Check sheet for the modelled part. Datum: model origin and axes. Units: mm. Face numbers are marked on the shaded views. A direction names the side the tool comes from. Give positions to 0.01 mm unless a question says otherwise; leave off trailing zeros. Write each loop counter-clockwise with the first axis right and the second up, starting at its lowest first coordinate (ties: lowest second). Pieces come first, ordered by that corner, then holes. Notation, with made-up numbers: M 83,89 L 131,89 A19 ccw 131,94 Z; hole C 17,51 d7. An arc over 180 degrees is marked long. Write item = value, one per line. Start each with the question number.
1) Sectioned sample at C-C, the plane z = 23. Record the cut outline in (x, y), then the cut area to 3 significant figures.
2) Gauge pin test, flat ends, axial feed: pin 1 (1 mm diameter, centred on y = 19, z = 24, fed in from +X); pin 2 (5 mm diameter, centred on x = 19, z = 14, fed in from +Y); pin 3 (10 mm diameter, centred on x = 25.5, z = 14.5, fed in from -Y). Record the tip position at first contact, or that the pin passes through.
3) Sectioned sample at A-A, the plane y = 1.75. Record the cut outline in (x, z).
4) Sectioned sample at D-D, the plane x = 2. Record the cut outline in (y, z).
5) Set-up check for the marked faces 1, 2 and 3: record each of +Z, -Z, +X, -X, +Y, -Y from which the full face is reachable in a straight line by a thin tool's end or side.
6) Draft check along X on the marked faces 4, 5 and 6. Enter one of: pulls with the +X half, pulls with the -X half, needs draft (parallel to the pull), parting line crosses it, or undercut.
7) Sectioned sample at B-B, the plane y = 8.75. Record the cut outline in (x, z), then the cut area to 3 significant figures.
8) Scan lines: L1, parallel to X at y = 13.5, z = 8.5; L2, parallel to X at y = 3.75, z = 3.5; L3, parallel to X at y = 19.75, z = 2. Record each from-to range of solid material in increasing order.
from build123d import *

# Parameters (mm, degrees)
F1_DEPTH    = 30
F2_T1_DEPTH = 55.7168298797


# Not quite as in the source:
# - a fillet or chamfer that OpenCascade refuses, or shapes differently, is made with other operations: its cross-section is extruded or revolved along the edge and cut away or added


with BuildPart() as f1:
    # F0 (on Top) → F1 (new body)
    with BuildSketch(Plane.XY):
        Polygon((-3.2, 0), (0, 0), (0, 20), (10, 20), (10, 0), (13.2, 0), (58.2, 0), (61.4, 0), (61.4, 19.8679156601), (58.2, 19.8679156601), (58.2, 4.00000019), (13.2, 4.00000019), (13.2, 23.2), (-3.2, 23.2), align=None)
    extrude(amount=F1_DEPTH)

    # F2: chamfer of 5 on 1 edges, made by hand

    # F2_s2 → F2_t1 (cut)
    with BuildSketch(Plane.XY.offset(-12.8584149398)):
        Polygon((56.4, 19.8679156601), (61.4, 14.8679156601), (61.4, 19.8679156601), align=None)
    extrude(amount=F2_T1_DEPTH, mode=Mode.SUBTRACT)


solid = f1.part
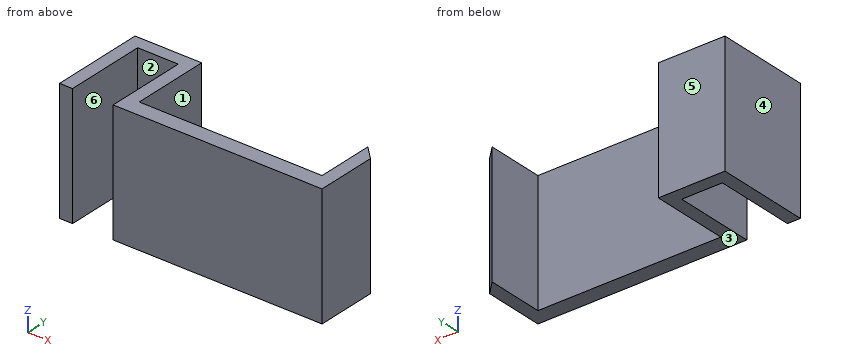
Data:
q1.outline = M -3.2,0 L 0,0 L 0,20 L 10,20 L 10,0 L 61.4,0 L 61.4,14.87 L 58.2,18.07 L 58.2,4 L 13.2,4 L 13.2,23.2 L -3.2,23.2 Z
q1.area = 413 mm2
q2.pin_1 = 13.2
q2.pin_2 = 4
q2.pin_3 = 0
q3.outline = M -3.2,0 L 0,0 L 0,30 L -3.2,30 Z; M 10,0 L 61.4,0 L 61.4,30 L 10,30 Z
q4.outline = M 20,0 L 23.2,0 L 23.2,30 L 20,30 Z
q5.face_1 = +Z, -Z, +Y
q5.face_2 = +Z, -Z, -Y
q5.face_3 = -Z, +X, -X, +Y, -Y
q6.face_4 = pulls with the -X half
q6.face_5 = needs draft
q6.face_6 = undercut
q7.outline = M -3.2,0 L 0,0 L 0,30 L -3.2,30 Z; M 10,0 L 13.2,0 L 13.2,30 L 10,30 Z; M 58.2,0 L 61.4,0 L 61.4,30 L 58.2,30 Z
q7.area = 288 mm2
q8.L1 = -3.2 to 0, 10 to 13.2, 58.2 to 61.4
q8.L2 = -3.2 to 0, 10 to 61.4
q8.L3 = -3.2 to 0, 10 to 13.2
